```python
from build123d import *

# Parameters (mm, degrees)
F0_R     = 24.5
F0_R_2   = 15
F0_R_3   = 10.5
F1_DEPTH = 24
F2_SIZE2 = 3
F2_SIZE  = 11
F0_R_4   = 29.5
F3_DEPTH = 16
F4_DEPTH = 5
F5_DEPTH = 5


# Not quite as in the source:
# - a feature names something its author has since deleted; it is built from what else it names


with BuildPart() as f1:
    # F0 (on Top) → F1 (new body)
    with BuildSketch(Plane.XY):
        Circle(F0_R)
        Circle(F0_R_2, mode=Mode.SUBTRACT)
        Circle(F0_R_2)
        Circle(F0_R_3, mode=Mode.SUBTRACT)
        Circle(F0_R_3)
    extrude(amount=-F1_DEPTH)

    # F2
    f2_edges = [f1.edges().sort_by_distance(p)[0] for p in [
        (-24.5, 0, -24),
    ]]
    f2_side = f1.faces().sort_by_distance((-24.5, 0, -12))[0]
    chamfer(f2_edges, length=F2_SIZE, length2=F2_SIZE2, reference=f2_side)

    # F0 (on Top) → F3 (cut)
    with BuildSketch(Plane.XY):
        Circle(F0_R_4)
        Circle(F0_R, mode=Mode.SUBTRACT)
        Circle(F0_R_2)
        Circle(F0_R_3, mode=Mode.SUBTRACT)
        Circle(F0_R_3)
    extrude(amount=-F3_DEPTH, mode=Mode.SUBTRACT)

    # F0 (on Top) → F4 (join)
    with BuildSketch(Plane.XY):
        Circle(F0_R_2)
        Circle(F0_R_3, mode=Mode.SUBTRACT)
    extrude(amount=-F4_DEPTH)

    # F0 (on Top) → F5 (join)
    with BuildSketch(Plane.XY):
        Circle(F0_R_4)
        Circle(F0_R, mode=Mode.SUBTRACT)
    extrude(amount=-F5_DEPTH)


solid = f1.part
```
Could you check a few things on this model? Use its own coordinates, in mm. A direction names the side the tool comes from. Coordinates: 2 decimals unless noted, no trailing zeros. Write each loop counter-clockwise with the first axis right and the second up, starting at its lowest first coordinate (ties: lowest second). Pieces come first, ordered by that corner, then holes. Notation, with made-up numbers: (76, 51) -> (88, 51) arc R17 cw to (88, 59) -> close; hole circle Ø2 at (-39.5, -39). An arc over 180 degrees is marked (long way). Return JSON: item names as keys, results as strings.
(1) Imagine slicing it at B-B, the plane y = 0. Please give me the cut outline in (x, z), then the cut area to 3 significant figures.
Numbers:
{"outline": "(-29.5, -5) -> (-24.5, -5) -> (-24.5, -13) -> (-21.5, -24) -> (21.5, -24) -> (24.5, -13) -> (24.5, -5) -> (29.5, -5) -> (29.5, 0) -> (10.5, 0) -> (10.5, -5) -> (15, -5) -> (15, -16) -> (-15, -16) -> (-15, -5) -> (-10.5, -5) -> (-10.5, 0) -> (-29.5, 0) -> close", "area": "758 mm2"}
(2) Which directions (+Z, -Z, +X, -X, +Y, -Y) give clear straight access to the entire face, cutting with the end or side of a thin tool? Please do faces 4 (the flat face through (3.1, 10.2, -5)), 5 (the cylindrical face through (10, 3.2, -2.5)), 6 (the flat face through (-7, 24, -5)), 7 (the flat face through (0, 0, -24)).
Numbers:
{"face 4": "none", "face 5": "+Z", "face 6": "-Z", "face 7": "-Z, +X, -X, +Y, -Y"}
(3) Imagine slicing it at D-D, the plane z = -21. Please give me the cut outline in (x, y), then the cut area to 3 significant figures.
Numbers:
{"outline": "circle Ø44.64 at (0, 0)", "area": "1,560 mm2"}
(4) I need wall thicknesses on L1, parallel to Y at x = 0, z = -11.25; L2, parallel to Z at x = -2, y = -14; L3, parallel to Y at x = 0, z = -3.8. Which ranges of each line are inside material? Lowest first, please.
Numbers:
{"L1": "y = -24.5 to -15, 15 to 24.5", "L2": "z = -24 to -16, -5 to 0", "L3": "y = -29.5 to -10.5, 10.5 to 29.5"}
(5) Imagine slicing it at A-A, the plane z = -12.25. Please give me the cut outline in (x, y).
Numbers:
{"outline": "circle Ø49 at (0, 0); hole circle Ø30 at (0, 0)"}
(6) I'm going to push flat-ended pins straight in: pin 1 (3 mm diameter, centred on y = -19.5, z = -18.5, fed in from -X); pin 2 (2 mm diameter, centred on x = 17, z = -10.5, fed in from +Y); pin 3 (18 mm diameter, centred on x = 0, y = 0, fed in from +Z). Where does each tip first touch, or does it pass through?
Numbers:
{"pin 1": "stops at x = -14.43", "pin 2": "stops at y = 18.55", "pin 3": "stops at z = -16"}
(7) We'd pull the mould along X, two halves only. Please class faces 1 (the cylindrical face through (13.17, 20.66, -8.94)), 2 (the flat face through (0, -13, 0)), 3 (the flat face through (0, 0, -16)): +X half, -X half, draft (parallel to the pull), parting line (faces both ways), or undercut.
Numbers:
{"face 1": "parting line", "face 2": "draft", "face 3": "undercut"}
